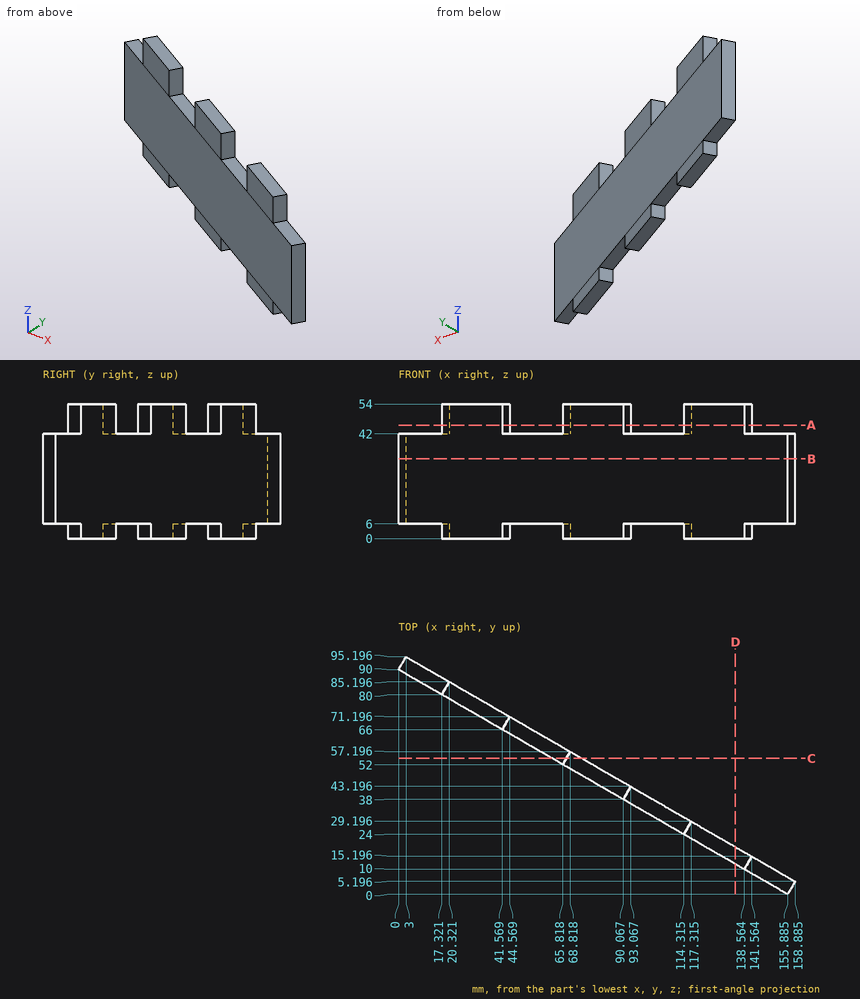
For this review, use the dimensioned drawing (mm, ordinates from the lowest corner) and the shaded views. Round coordinates to 2 decimals unless told otherwise and drop trailing zeros. Write each loop counter-clockwise with the first axis right and the second up, starting at its lowest first coordinate (ties: lowest second). Pieces come first, ordered by that corner, then holes. Notation, with made-up numbers: (39, 22.5) -> (68, 22.5) arc R10 ccw to (68, 31.5) -> close; hole circle Ø3 at (40, -10). An arc over 180 degrees is marked (long way). Use CSV: the item, a comma, the result in double quotes.
(1) Consider section D-D, the plane x = 135. Give the boundary of the cut face in (y, z) (1 decimal), plus the area to 3 significant figures.
Computed values:
outline,"(12.1, 0) -> (19, 0) -> (19, 54) -> (12.1, 54) -> close"
area,"374 mm²"
(2) Consider section C-C, the plane y = 54.5. Give the boundary of the cut face in (x, z).
Computed values:
outline,"(61.49, 6) -> (67.26, 6) -> (67.26, 0) -> (73.49, 0) -> (73.49, 54) -> (67.26, 54) -> (67.26, 42) -> (61.49, 42) -> close"
(3) To check wall thickness, follow L1, parallel to X at y = 15.5, z = 11 (1 decimal); L2, parallel to X at y = 66.5, z = 47.5 (1 decimal); L3, parallel to Y at x = 92.5, z = 36 (1 decimal). State the ranges of each line that lie inside material, in increasing order. Write a range as [from, to].
Computed values:
L1,"[129, 141]"
L2,"[40.7, 41.9]"
L3,"[36.6, 43.5]"
(4) Clearance check with flat-ended pins moving along their axes: P1, Ø8, axis at x = 135.5, z = 11, coming from the -Y side; P2, Ø4.5, axis at x = 144.5, y = 6, coming from the -Z side; P3, Ø6, axis at x = 52.5, y = 63, coming from the +Z side. State where each tip first meets the part, or that it passes through.
Computed values:
P1,"y = 9.46"
P2,"z = 6"
P3,"z = 42"
(5) Consider section B-B, the plane z = 32. Give the boundary of the cut face in (x, y) (1 decimal), plus the area to 3 significant figures.
Computed values:
outline,"(0, 90) -> (155.9, 0) -> (158.9, 5.2) -> (3, 95.2) -> close"
area,"1,080 mm²"
(6) Consider section A-A, the plane z = 45.5. Give the boundary of the cut face in (x, y) (1 decimal), plus the area to 3 significant figures.
Computed values:
outline,"(17.3, 80) -> (41.6, 66) -> (44.6, 71.2) -> (20.3, 85.2) -> close; (65.8, 52) -> (90.1, 38) -> (93.1, 43.2) -> (68.8, 57.2) -> close; (114.3, 24) -> (138.6, 10) -> (141.6, 15.2) -> (117.3, 29.2) -> close"
area,"504 mm²"
